The listing builds one solid part. Answer for the finished solid, in the listing's coordinates (mm). A direction names the side the tool comes from. Coordinates: 2 decimals unless noted, no trailing zeros. Loops run counter-clockwise (first coordinate to the right, second up) from the corner with the lowest first, then second, coordinate; pieces in that order, holes last. Notation, with made-up numbers: (61, 74.25) - (101, 74.25) arc R7 cw to (101, 81.25) - close; hole circle Ø8 at (-32, 39.5). An arc over 180 degrees is marked (long way). Write each question's results on one line, items separated by ' | '. Start each with the question number.
(1) Find section C-C on z = 7. Determine the outline of the cut face in (x, y).
(2) Determine the mould class of faces 5 (the cylindrical face through (11.967, 7.47, 5.765)), 6 (the flat face through (9, 12.54, 6)), 7 (the cylindrical face through (0.06, 0.04, 5.75)), 8 (the flat face through (5.83, 0.04, 5.1)) for opening direction Z: released by +Z, released by -Z, zero draft, split by the parting line, or undercut.
(3) Find section B-B on z = 0. Determine the outline of the cut face in (x, y), then the cut area to 3 significant figures.
(4) Consider line 1 (X direction, y = 0, z = 0); line 2 (X direction, y = 1.25, z = -1); line 3 (X direction, y = -2.25, z = 3). Determine where each line is inside the solid, lowest interval first. Write a range as from..to.
(5) Find section A-A on x = 0. Determine the outline of the cut face in (y, z).
(6) Given pin 1 Ø1.5 at (x, z) = (-9, -12.5) entering from +Y; pin 2 Ø4.5 at (y, z) = (-0.5, -7.5) entering from -X; pin 3 Ø2.5 at (x, z) = (-1.5, -1) entering from +Y, each flat-ended and moving along its own axis, determine where each tip first touches the part or whether it passes through.
(7) Find section D-D on y = 1. State how many separate pieces and enclosed holes the cut face has, then the cut area to 3 significant figures.
(8) For faces 1 (the cylindrical face through (-8.97, 0.04, -8.99)), 2 (the cylindrical face through (13.967, 0.036, 6.041)), 3 (the cylindrical face through (-6.1, 0.04, -14.02)), 4 (the cylindrical face through (-15.188, 0.036, -1.727)), determine the directions among +Z, -Z, +X, -X, +Y, -Y from which every point of the face is accessible in a straight line to the end or side of a thin tool.
from build123d import *

# Parameters (mm, degrees)
BASE_PROFILE_R          = 12.7
GEAR_BASE_DEPTH         = 2.54
GEAR_START              = 2.54
GEAR_TOOTH_DEPTH        = 5.08
PATTERN_TOOTH_12T_COUNT = 12
LIP_PROFILE_R           = 4.348362351
LIP_DEPTH               = 3.5
SHAFT_START             = 0.96
HOLE_PROFILE_R          = 2.75
SHAFT_HOLE_DEPTH        = 7
GEAR_CUTOUT_DEPTH       = 5.08
HANDLE_PROFILE_R        = 2.5
HANDLE_DEPTH            = 10


with BuildPart() as part:
    # Base Profile → Gear Base (new, symmetric)
    with BuildSketch(Plane(origin=(0, 0, 0), x_dir=(1, 0, 0), z_dir=(0, 1, 0))):
        with Locations(Location((0, 0, 0), (0, 0, 270))):
            Circle(BASE_PROFILE_R)
    extrude(amount=GEAR_BASE_DEPTH, both=True)

    # Tooth Profile → Gear Tooth (add)
    with BuildSketch(Plane(origin=(0, 0, 0), x_dir=(1, 0, 0), z_dir=(0, 1, 0)).offset(GEAR_START)):
        with BuildLine():
            ThreePointArc((-2.286, 12.492565949), (-1.739501602, 15.15244151), (-0.508, 17.572565949))
            ThreePointArc((-0.508, 17.572565949), (0, 17.576799577), (0.508, 17.572565949))
            ThreePointArc((0.508, 17.572565949), (1.739501602, 15.15244151), (2.286, 12.492565949))
            ThreePointArc((2.286, 12.492565949), (0, 12.7), (-2.286, 12.492565949))
        make_face()
    gear_tooth = extrude(amount=-GEAR_TOOTH_DEPTH)

    # Pattern Tooth (12T): Gear Tooth ×12 about axis
    pattern_tooth_12t_axis = Axis((0, 0, 0), (0, 1, 0))
    for i in range(1, PATTERN_TOOTH_12T_COUNT):
        add(gear_tooth.rotate(pattern_tooth_12t_axis, i * 360 / PATTERN_TOOTH_12T_COUNT))

    # Lip Profile → Lip (add, symmetric)
    with BuildSketch(Plane(origin=(0, 0, 0), x_dir=(1, 0, 0), z_dir=(0, 1, 0))):
        with Locations(Location((0, 0, 0), (0, 0, 270))):
            Circle(LIP_PROFILE_R)
    extrude(amount=LIP_DEPTH, both=True)

    # Hole Profile → Shaft Hole (cut)
    with BuildSketch(Plane(origin=(0, 2.54, 0), x_dir=(1, 0, 0), z_dir=(0, 1, 0)).offset(SHAFT_START)):
        with Locations(Location((0, 0, 0), (0, 0, 270))):
            Circle(HOLE_PROFILE_R)
    extrude(amount=-SHAFT_HOLE_DEPTH, mode=Mode.SUBTRACT)

    # Cutout Profile → Gear Cutout (cut)
    with BuildSketch(Plane(origin=(0, 2.54, 0), x_dir=(1, 0, 0), z_dir=(0, 1, 0))):
        with BuildLine():
            Line((-1.5, 9.583318841), (-1.5, 5.550900828))
            ThreePointArc((-1.5, 5.550900828), (-4.979646072, 2.875), (-5.557221131, -1.476412308))
            Line((-5.557221131, -1.476412308), (-9.049397568, -3.492621315))
            ThreePointArc((-9.049397568, -3.492621315), (-8.400446417, 4.85), (-1.5, 9.583318841))
        make_face()
        with BuildLine():
            Line((1.5, 9.583318841), (1.5, 5.550900828))
            ThreePointArc((1.5, 5.550900828), (4.979646072, 2.875), (5.557221131, -1.476412308))
            Line((5.557221131, -1.476412308), (9.049397568, -3.492621315))
            ThreePointArc((9.049397568, -3.492621315), (8.400446417, 4.85), (1.5, 9.583318841))
        make_face()
        with BuildLine():
            Line((7.549397568, -6.090697526), (4.057221131, -4.07448852))
            ThreePointArc((4.057221131, -4.07448852), (0, -5.75), (-4.057221131, -4.07448852))
            Line((-4.057221131, -4.07448852), (-7.549397568, -6.090697526))
            ThreePointArc((-7.549397568, -6.090697526), (0, -9.7), (7.549397568, -6.090697526))
        make_face()
    extrude(amount=-GEAR_CUTOUT_DEPTH, mode=Mode.SUBTRACT)

    # Handle Profile → Handle (add)
    with BuildSketch(Plane(origin=(0, 2.54, 0), x_dir=(1, 0, 0), z_dir=(0, 1, 0))):
        with Locations(Location((9.483758311, -5.475450414, 0), (0, 0, 95.868617156))):
            Circle(HANDLE_PROFILE_R)
    extrude(amount=HANDLE_DEPTH)


solid = part.part
Values:
1) outline: (-14.7, -2.54) - (-6.71, -2.54) - (-6.71, 2.54) - (-14.7, 2.54) - close; (6.71, -2.54) - (14.7, -2.54) - (14.7, 2.54) - (11.47, 2.54) - (11.47, 12.54) - (7.5, 12.54) - (7.5, 2.54) - (6.71, 2.54) - close
2) face 5: split by the parting line | face 6: zero draft | face 7: undercut | face 8: undercut
3) outline: (-17.58, -2.54) - (-9.7, -2.54) - (-9.7, 2.54) - (-17.58, 2.54) - close; (-5.75, -2.54) - (-4.35, -2.54) - (-4.35, -3.5) - (-2.75, -3.5) - (-2.75, 3.5) - (-4.35, 3.5) - (-4.35, 2.54) - (-5.75, 2.54) - close; (2.75, -3.5) - (4.35, -3.5) - (4.35, -2.54) - (5.75, -2.54) - (5.75, 2.54) - (4.35, 2.54) - (4.35, 3.5) - (2.75, 3.5) - close; (9.7, -2.54) - (17.58, -2.54) - (17.58, 2.54) - (9.7, 2.54) - close | area: 117 mm²
4) line 1: x = -17.58..-9.7, -5.75..-2.75, 2.75..5.75, 9.7..17.58 | line 2: x = -16.79..-9.65, -5.66..-2.56, 2.56..5.66, 9.65..16.79 | line 3: x = -12.34..-9.22, -8.2..8.2, 9.22..12.34
5) outline: (-3.5, -4.35) - (-2.54, -4.35) - (-2.54, -17.58) - (2.54, -17.58) - (2.54, -4.35) - (3.5, -4.35) - (3.5, -2.75) - (-3.5, -2.75) - close; (-3.5, 2.75) - (3.5, 2.75) - (3.5, 4.35) - (2.54, 4.35) - (2.54, 5.75) - (-2.54, 5.75) - (-2.54, 4.35) - (-3.5, 4.35) - close; (-2.54, 9.7) - (2.54, 9.7) - (2.54, 17.58) - (-2.54, 17.58) - close
6) pin 1: stops at y = 2.54 | pin 2: stops at x = -15.47 | pin 3: stops at y = 3.5
7) separate pieces: 1 | enclosed holes: 4 | area: 521 mm²
8) face 1: +Y, -Y | face 2: +X, +Y, -Y | face 3: -Z, +Y, -Y | face 4: -X, +Y, -Y
